For this review, take the finished solid that the model builds, in its own axes (mm). Face numbers are marked on the shaded views. A direction names the side the tool comes from. Coordinates: 2 decimals unless noted, no trailing zeros. Order: outer loops, then holes, each group sorted by start corner. A loop starts at its lowest first (then second) coordinate and runs counter-clockwise, first axis right, second up. Notation, with made-up numbers: (-2.75, -22) - (28.25, -22) arc R8 ccw to (28.25, -15) - close; hole circle Ø9 at (-37.75, -25.5). An arc over 180 degrees is marked (long way). One line per item, written item: value. Start each with the question number.
(1) Consider section C-C on x = 28. Write out the cut boundary in (y, z), then the cut area to 3 significant figures.
(2) Consider section A-A on y = 0. Write out the cut boundary in (x, z).
(3) Clearance check with flat-ended pins moving along their axes: pin 1 (2 mm diameter, centred on y = 3, z = 5.2, fed in from +X); pin 2 (6 mm diameter, centred on x = 25.5, y = -5, fed in from +Z); pin 3 (6 mm diameter, centred on x = 15, y = -6, fed in from +Z). State where each tip first meets the part, or that it passes through.
(4) Consider section D-D on y = -5.5. Write out the cut boundary in (x, z), then the cut area to 3 significant figures.
(5) Consider section B-B on z = 0. Write out the cut boundary in (x, y), then the cut area to 3 significant figures.
(6) To check wall thickness, follow line 1 along X through (y, z) = (-5.5, 1.5); line 2 along X through (y, z) = (-2, 5.75); line 3 along Y through (x, z) = (17, -8.25). State the ranges of each line that lie inside material, in increasing order.
(7) For the marked faces 1 and 2, list the 3-axis set-ups (+Z, -Z, +X, -X, +Y, -Y) from which the entire face can be reached by the end or side of a thin tool; tool diameter is ignored.
```python
from build123d import *

# Parameters (mm, degrees)
CROQUIS4_R              = 10
SALIENTE_EXTRUIR2_DEPTH = 25
CROQUIS5_R              = 3
SALIENTE_EXTRUIR3_DEPTH = 1.5
CROQUIS6_R              = 1.5
SALIENTE_EXTRUIR4_DEPTH = 0.5
CROQUIS7_R              = 1
SALIENTE_EXTRUIR5_DEPTH = 6
REDONDEO1_R             = 1
CROQUIS10_R             = 9.905946753
SALIENTE_EXTRUIR6_DEPTH = 1
CORTAR_EXTRUIR1_START   = 1
CROQUIS8_R              = 1.25
CORTAR_EXTRUIR1_DEPTH   = 6


with BuildPart() as part:
    # Croquis4 → Saliente-Extruir2 (new body)
    with BuildSketch(Plane(origin=(0, 0, 0), x_dir=(0, 0, -1), z_dir=(1, 0, 0))):
        Circle(CROQUIS4_R)
    extrude(amount=SALIENTE_EXTRUIR2_DEPTH)

    # Croquis5 → Saliente-Extruir3 (add)
    with BuildSketch(Plane(origin=(25, 0, 0), x_dir=(0, 0, -1), z_dir=(1, 0, 0))):
        Circle(CROQUIS5_R)
    extrude(amount=SALIENTE_EXTRUIR3_DEPTH)

    # Croquis6 → Saliente-Extruir4 (add)
    with BuildSketch(Plane(origin=(26.5, 0, 0), x_dir=(0, 0, -1), z_dir=(1, 0, 0))):
        Circle(CROQUIS6_R)
    extrude(amount=SALIENTE_EXTRUIR4_DEPTH)

    # Croquis7 → Saliente-Extruir5 (add)
    with BuildSketch(Plane(origin=(27, 0, 0), x_dir=(0, 0, -1), z_dir=(1, 0, 0))):
        Circle(CROQUIS7_R)
    extrude(amount=SALIENTE_EXTRUIR5_DEPTH)

    # Redondeo1
    redondeo1_edges = [part.edges().sort_by_distance(p)[0] for p in [
        (33, 0, 1),
    ]]
    fillet(redondeo1_edges, radius=REDONDEO1_R)

    # Croquis10 → Saliente-Extruir6 (add)
    with BuildSketch(Plane(origin=(25, 0, 0), x_dir=(0, 0, -1), z_dir=(1, 0, 0))):
        Circle(CROQUIS10_R)
    extrude(amount=SALIENTE_EXTRUIR6_DEPTH)

    # Croquis8 → Cortar-Extruir1 (cut)
    with BuildSketch(Plane(origin=(25, 0, 0), x_dir=(0, 0, -1), z_dir=(1, 0, 0)).offset(CORTAR_EXTRUIR1_START)):
        with Locations((0, 6)):
            Circle(CROQUIS8_R)
        with Locations((5.196152423, 3)):
            Circle(CROQUIS8_R)
        with Locations((5.196152423, -3)):
            Circle(CROQUIS8_R)
        with Locations((0, -6)):
            Circle(CROQUIS8_R)
        with Locations((-5.196152423, -3)):
            Circle(CROQUIS8_R)
        with Locations((-5.196152423, 3)):
            Circle(CROQUIS8_R)
    extrude(amount=-CORTAR_EXTRUIR1_DEPTH, mode=Mode.SUBTRACT)


solid = part.part
```
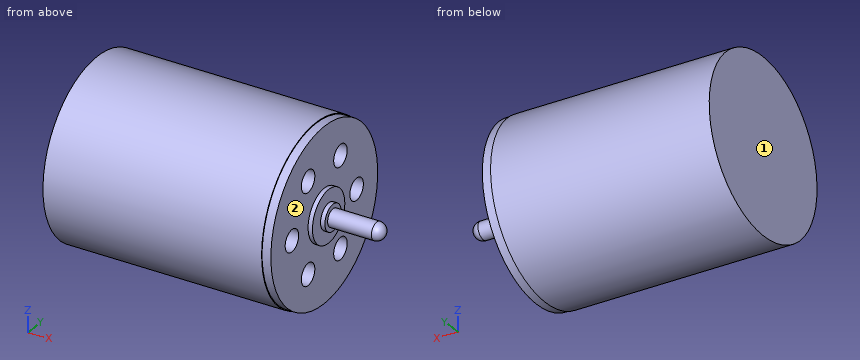
Geometry check:
1. outline: circle Ø2 at (0, 0)
1. area: 3.14 mm^2
2. outline: (0, -10) - (25, -10) - (25, -9.91) - (26, -9.91) - (26, -3) - (26.5, -3) - (26.5, -1.5) - (27, -1.5) - (27, -1) - (32, -1) arc R1 ccw to (32, 1) - (27, 1) - (27, 1.5) - (26.5, 1.5) - (26.5, 3) - (26, 3) - (26, 9.91) - (25, 9.91) - (25, 10) - (0, 10) - close
3. pin 1: stops at x = 20
3. pin 2: stops at z = 9.79
3. pin 3: stops at z = 9.54
4. outline: (0, -8.35) - (25, -8.35) - (25, -8.24) - (26, -8.24) - (26, -1.15) - (20, -1.15) - (20, 1.15) - (26, 1.15) - (26, 8.24) - (25, 8.24) - (25, 8.35) - (0, 8.35) - close
4. area: 420 mm^2
5. outline: (0, -10) - (25, -10) - (25, -9.91) - (26, -9.91) - (26, -7.25) - (20, -7.25) - (20, -4.75) - (26, -4.75) - (26, -3) - (26.5, -3) - (26.5, -1.5) - (27, -1.5) - (27, -1) - (32, -1) arc R1 ccw to (32, 1) - (27, 1) - (27, 1.5) - (26.5, 1.5) - (26.5, 3) - (26, 3) - (26, 4.75) - (20, 4.75) - (20, 7.25) - (26, 7.25) - (26, 9.91) - (25, 9.91) - (25, 10) - (0, 10) - close
5. area: 506 mm^2
6. line 1: x = 0 to 26
6. line 2: x = 0 to 20
6. line 3: y = -5.65 to 5.65
7. face 1: +Z, -Z, -X, +Y, -Y
7. face 2: +X
